Input: part model. Units: mm. Frame: model coordinates. A direction names the side the tool comes from. Round coordinates to 2 decimals unless told otherwise and drop trailing zeros. Loops run counter-clockwise (first coordinate to the right, second up) from the corner with the lowest first, then second, coordinate; pieces in that order, holes last.
1) First-contact query: pin 1 (12 mm diameter, centred on x = 22.5, z = 14, fed in from -Y); pin 2 (3.5 mm diameter, centred on x = -10, z = 15, fed in from +Y); pin 3 (5.5 mm diameter, centred on x = -27.5, z = 14.5, fed in from -Y); pin 4 (1.5 mm diameter, centred on x = 26.5, y = 5, fed in from -Z). Flat tips, straight axial feed; report the tip coordinate or a pass-through.
2) Draft query along Z for faces 1 (the face through (8.492, 6.678, 1.719)), 2 (the face through (39.235, 0.474, 15.012)), 3 (the face through (-19.547, -1.549, 15.716)). Return one class per face: pulls with the +Z half, pulls with the -Z half, needs draft (parallel to the pull), parting line crosses it, or undercut.
3) Access query for faces 4 (the face through (-12.867, 8.114, 2.218)), 5 (the face through (1.02, -1.33, 7.33)), 6 (the face through (22.6, 2, 15.1)), 7 (the face through (-19, -5, 15)). Directions: +Z, -Z, +X, -X, +Y, -Y. A direction counts if a zero-diameter tool reaches every point of the face in a straight line with its end or side. Return the directions, or none.
4) Section B-B, the plane y = 0. State how many separate pieces and enclosed holes the cut face has, and give its area (3 significant figures).
5) Ray query, line 1 along X through (y, z) = (0.5, 27.5); line 2 along Z through (x, y) = (10, -3.25); line 3 along Y through (x, z) = (50, 7.5) (3 decimals). Return the intervals inside material, ascending.
6) Section A-A, the plane x = -25. Return loops of the section in (y, z), and give its area (3 significant figures).
7) Section C-C, the plane x = 0. Return loops of the section in (y, z) (3 decimals), and give its area (3 significant figures).
8) Section D-D, the plane z = 24. Return loops of the section in (x, y) (3 decimals), and give its area (3 significant figures).
from build123d import *
from OCP.BRepFilletAPI import BRepFilletAPI_MakeChamfer

# Parameters (mm, degrees)
SKETCH1_R                     = 10.775
SKETCH1_W                     = 7
SKETCH1_H                     = 1.9
BOSS_EXTRUDE1_DEPTH           = 30
BOSS_EXTRUDE4_DEPTH           = 5
BOSS_EXTRUDE4_DEPTH_BACK      = 5
SKETCH30_R                    = 1.675
CUT_EXTRUDE14_DEPTH           = 75.167487823
SKETCH31_R                    = 4
CUT_EXTRUDE15_DEPTH           = 2.2
CHAMFER1_SIZE                 = 1
SKETCH42_W                    = 10.885616931
SKETCH42_H                    = 7.232184452
BOSS_EXTRUDE6_DEPTH           = 4.5
BOSS_EXTRUDE6_DRAFT           = -30
BOSS_EXTRUDE6_PROFILE_2_DEPTH = 4.5
BOSS_EXTRUDE6_PROFILE_2_DRAFT = -30
CUT_EXTRUDE16_DEPTH           = 73.897882342
CUT_EXTRUDE16_DEPTH_BACK      = 73.897882342
SKETCH43_R                    = 1.95
SKETCH43_R_2                  = 1.5
CHAMFER2_SIZE                 = 0.5
CHAMFER3_SIZE                 = 1
CHAMFER3_SIZE2                = 0.577350269
SKETCH44_R                    = 5.5
CUT_EXTRUDE17_DEPTH           = 7


with BuildPart() as part:
    # Sketch1 → Boss-Extrude1 (new body)
    with BuildSketch(Plane.XY):
        with BuildLine():
            Line((-33.091348368, 2.425), (33.073098334, 2.425))
            ThreePointArc((33.073098334, 2.425), (34.841312767, 3.001486492), (35.929959375, 4.509388186))
            ThreePointArc((35.929959375, 4.509388186), (64.775, 0), (35.929959375, -4.509388186))
            ThreePointArc((35.929959375, -4.509388186), (34.841312767, -3.001486492), (33.073098334, -2.425))
            Line((33.073098334, -2.425), (12.362013388, -2.425))
            ThreePointArc((12.362013388, -2.425), (10.721383427, -2.913360429), (9.614899302, -4.219444444))
            ThreePointArc((9.614899302, -4.219444444), (-0.006360753, -10.499998073), (-9.620004404, -4.207792208))
            ThreePointArc((-9.620004404, -4.207792208), (-10.717205737, -2.910276804), (-12.345672319, -2.425))
            Line((-12.345672319, -2.425), (-33.091348368, -2.425))
            ThreePointArc((-33.091348368, -2.425), (-34.84606209, -2.99758356), (-35.925333642, -4.494929577))
            ThreePointArc((-35.925333642, -4.494929577), (-64.775, 0), (-35.925333642, 4.494929577))
            ThreePointArc((-35.925333642, 4.494929577), (-34.84606209, 2.99758356), (-33.091348368, 2.425))
        make_face()
        with Locations((50, 0)):
            Circle(SKETCH1_R, mode=Mode.SUBTRACT)
        with Locations(Location((-50, 0, 0), (0, 0, 180))):
            Circle(SKETCH1_R, mode=Mode.SUBTRACT)
        with Locations((0, -6.3)):
            Rectangle(SKETCH1_W, SKETCH1_H, mode=Mode.SUBTRACT)
    extrude(amount=BOSS_EXTRUDE1_DEPTH)

    # Sketch32 → Boss-Extrude4 (add, two sides: drawn at the far end of the back side and taken through both)
    with BuildSketch(Plane.XZ.offset(-BOSS_EXTRUDE4_DEPTH_BACK)):
        Polygon((-38.661098901, 30), (7.988715583, 30), (38.752094408, 30), (38.752094408, 0), (7.988715583, 0), (-38.661098901, 0), align=None)
    extrude(amount=BOSS_EXTRUDE4_DEPTH + BOSS_EXTRUDE4_DEPTH_BACK)

    # Sketch30 → Cut-Extrude14 (cut, through all)
    with BuildSketch(Plane(origin=(0, -5.35, 0), x_dir=(1, 0, 0), z_dir=(0, 1, 0))):
        with Locations(Location((0, -6, 0), (0, 0, 90))):
            Circle(SKETCH30_R)
        with Locations(Location((0, -24, 0), (0, 0, 90))):
            Circle(SKETCH30_R)
    extrude(amount=CUT_EXTRUDE14_DEPTH, mode=Mode.SUBTRACT)

    # Sketch31 → Cut-Extrude15 (cut)
    with BuildSketch(Plane(origin=(0, 5, 0), x_dir=(1, 0, 0), z_dir=(0, 1, 0))):
        with Locations(Location((0, -6, 0), (0, 0, 270))):
            Circle(SKETCH31_R)
        with Locations(Location((0, -24, 0), (0, 0, 270))):
            Circle(SKETCH31_R)
    extrude(amount=-CUT_EXTRUDE15_DEPTH, mode=Mode.SUBTRACT)

    # Chamfer1
    chamfer1_edges = [part.edges().sort_by_distance(p)[0] for p in [
        (0, -5.35, 0),
        (0, -5.35, 30),
    ]]
    chamfer(chamfer1_edges, length=CHAMFER1_SIZE)


with BuildPart() as boss_extrude6_tool:
    # Sketch42 → Boss-Extrude6 (with draft: the straight prism first)
    with BuildSketch(Plane(origin=(0, 0, 0), x_dir=(-1, 0, 0), z_dir=(0, 0, -1))):
        with Locations((-12.942808466, 5.778527688)):
            Rectangle(SKETCH42_W, SKETCH42_H)
    extrude(amount=-BOSS_EXTRUDE6_DEPTH)
    # Boss-Extrude6: the draft: its side faces are tilted about the plane it starts from
    boss_extrude6_sides = [boss_extrude6_tool.faces().sort_by_distance(p)[0] for p in [
        (7.5, 5.778527688, 2.25),
        (12.942808466, 9.394619914, 2.25),
        (18.385616931, 5.778527688, 2.25),
        (12.942808466, 2.162435462, 2.25),
    ]]
    draft(boss_extrude6_sides, Plane(origin=(0, 0, 0), x_dir=(-1, 0, 0), z_dir=(0, 0, -1)), BOSS_EXTRUDE6_DRAFT)


with BuildPart() as part_1:
    add(part.part)

    # Boss-Extrude6: add boss_extrude6_tool
    add(boss_extrude6_tool.part)


with BuildPart() as boss_extrude6_profile_2_tool:
    # Sketch42 → Boss-Extrude6 profile 2 (with draft: the straight prism first)
    with BuildSketch(Plane(origin=(0, 0, 0), x_dir=(-1, 0, 0), z_dir=(0, 0, -1))):
        with Locations((12.942808466, 5.778527688)):
            Rectangle(SKETCH42_W, SKETCH42_H)
    extrude(amount=-BOSS_EXTRUDE6_PROFILE_2_DEPTH)
    # Boss-Extrude6 profile 2: the draft: its side faces are tilted about the plane it starts from
    boss_extrude6_profile_2_sides = [boss_extrude6_profile_2_tool.faces().sort_by_distance(p)[0] for p in [
        (-18.385616931, 5.778527688, 2.25),
        (-12.942808466, 9.394619914, 2.25),
        (-7.5, 5.778527688, 2.25),
        (-12.942808466, 2.162435462, 2.25),
    ]]
    draft(boss_extrude6_profile_2_sides, Plane(origin=(0, 0, 0), x_dir=(-1, 0, 0), z_dir=(0, 0, -1)), BOSS_EXTRUDE6_PROFILE_2_DRAFT)


with BuildPart() as part_2:
    add(part_1.part)

    # Boss-Extrude6 profile 2: add boss_extrude6_profile_2_tool
    add(boss_extrude6_profile_2_tool.part)

    # Sketch43 → Cut-Extrude16 (cut, two sides: drawn at the far end of the back side and taken through both)
    with BuildSketch(Plane(origin=(0, 0, 0), x_dir=(1, 0, 0), z_dir=(0, 1, 0)).offset(-CUT_EXTRUDE16_DEPTH_BACK)):
        with Locations(Location((25, -15, 0), (0, 0, 270))):
            Circle(SKETCH43_R)
        with Locations(Location((-25, -15, 0), (0, 0, 270))):
            Circle(SKETCH43_R)
        with Locations(Location((10, -15, 0), (0, 0, 239.251434948))):
            Circle(SKETCH43_R_2)
        with Locations(Location((-10, -15, 0), (0, 0, 300.748565052))):
            Circle(SKETCH43_R_2)
    extrude(amount=CUT_EXTRUDE16_DEPTH + CUT_EXTRUDE16_DEPTH_BACK, mode=Mode.SUBTRACT)

    # Chamfer2
    chamfer2_edges = [part_2.edges().sort_by_distance(p)[0] for p in [
        (25, 5, 13.05),
        (-25, 5, 13.05),
    ]]
    chamfer(chamfer2_edges, length=CHAMFER2_SIZE)

    # Chamfer3: one chamfer whose edges measure the first distance from different faces: ONE call of the kernel's chamfer builder (chamfer() names one face for all edges)
    chamfer3_edges_1 = [part_2.edges().sort_by_distance(p)[0] for p in [
        (39.225, 0, 0),
    ]]
    chamfer3_side_1 = [part_2.faces().sort_by_distance(p)[0] for p in [
        (39.225, 0, 15),
    ]]
    chamfer3_edges_2 = [part_2.edges().sort_by_distance(p)[0] for p in [
        (39.225, 0, 30),
        (-39.225, 0, 30),
    ]]
    chamfer3_side_2 = [part_2.faces().sort_by_distance(p)[0] for p in [
        (0, -0.289813178, 30),
    ]]
    chamfer3_edges_3 = [part_2.edges().sort_by_distance(p)[0] for p in [
        (-39.225, 0, 0),
    ]]
    chamfer3_side_3 = [part_2.faces().sort_by_distance(p)[0] for p in [
        (-39.225, 0, 15),
    ]]
    chamfer3 = BRepFilletAPI_MakeChamfer(part_2.part.solid().wrapped)
    for e in chamfer3_edges_1:
        chamfer3.Add(CHAMFER3_SIZE, CHAMFER3_SIZE2, e.wrapped, chamfer3_side_1[0].wrapped)  # the first distance lies on this face
    for e in chamfer3_edges_2:
        chamfer3.Add(CHAMFER3_SIZE, CHAMFER3_SIZE2, e.wrapped, chamfer3_side_2[0].wrapped)  # the first distance lies on this face
    for e in chamfer3_edges_3:
        chamfer3.Add(CHAMFER3_SIZE, CHAMFER3_SIZE2, e.wrapped, chamfer3_side_3[0].wrapped)  # the first distance lies on this face
    add(Compound.cast(chamfer3.Shape()), mode=Mode.REPLACE)

    # Sketch44 → Cut-Extrude17 (cut)
    with BuildSketch(Plane.XZ.offset(5)):
        with Locations(Location((25, 15, 0), (0, 0, 270))):
            Circle(SKETCH44_R)
        with Locations(Location((-25, 15, 0), (0, 0, 270))):
            Circle(SKETCH44_R)
    extrude(amount=-CUT_EXTRUDE17_DEPTH, mode=Mode.SUBTRACT)


solid = part_2.part
Final values:
1. pin 1: stops at y = -5
1. pin 2: stops at y = 5
1. pin 3: stops at y = 2
1. pin 4: stops at z = 0
2. face 1: pulls with the +Z half
2. face 2: needs draft
2. face 3: undercut
3. face 4: +Z, +Y
3. face 5: +Y
3. face 6: -Y
3. face 7: +Z, -Z, -Y
4. separate pieces: 3
4. enclosed holes: 6
4. area: 2,370 mm2
5. line 1: x = -64.77 to -60.76, -39.24 to 39.24, 60.76 to 64.77
5. line 2: z = 0 to 13.5, 16.5 to 30
5. line 3: y = -14.775 to -10.775, 10.775 to 14.775
6. outline: (-5, 0) - (5, 0) - (5, 12.55) - (4.5, 13.05) - (2, 13.05) - (2, 9.5) - (-5, 9.5) - close; (-5, 20.5) - (2, 20.5) - (2, 16.95) - (4.5, 16.95) - (5, 17.45) - (5, 30) - (-5, 30) - close
6. area: 211 mm2
7. outline: (-10.5, 0) - (-7.25, 0) - (-7.25, 30) - (-10.5, 30) - close; (-5.35, 1) - (-4.35, 0) - (5, 0) - (5, 2) - (2.8, 2) - (2.8, 4.325) - (-5.35, 4.325) - close; (-5.35, 7.675) - (2.8, 7.675) - (2.8, 10) - (5, 10) - (5, 20) - (2.8, 20) - (2.8, 22.325) - (-5.35, 22.325) - close; (-5.35, 25.675) - (2.8, 25.675) - (2.8, 28) - (5, 28) - (5, 30) - (-4.35, 30) - (-5.35, 29) - close
7. area: 317 mm2
8. outline: (-36.097, -5) - (-9.233, -5) arc R10.5 ccw to (9.233, -5) - (36.097, -5) arc R14.775 ccw (long way) to (36.097, 5) - (4, 5) - (4, 2.8) - (1.675, 2.8) - (1.675, -5.35) - (3.5, -5.35) - (3.5, -7.25) - (-3.5, -7.25) - (-3.5, -5.35) - (-1.675, -5.35) - (-1.675, 2.8) - (-4, 2.8) - (-4, 5) - (-36.097, 5) arc R14.775 ccw (long way) to start; hole circle Ø21.55 at (-50, 0); hole circle Ø21.55 at (50, 0)
8. area: 1,370 mm2
